Part model, mm, in its own coordinate system. Coordinates: 2 decimals unless noted, no trailing zeros. Order: outer loops, then holes, each group sorted by start corner. A loop starts at its lowest first (then second) coordinate and runs counter-clockwise, first axis right, second up.
from build123d import *

# Parameters (mm, degrees)
SKETCH1_W           = 6.35
SKETCH1_H           = 76.2
BOSS_EXTRUDE1_DEPTH = 114.3
SKETCH2_W           = 6.35
SKETCH2_H           = 50.8
BOSS_EXTRUDE2_DEPTH = 6.35
SKETCH3_W           = 6.35
SKETCH3_H           = 12.7
SKETCH3_W_2         = 95.25
SKETCH3_H_2         = 6.35
SKETCH3_W_3         = 25.4
CUT_EXTRUDE1_DEPTH  = 121.65


with BuildPart() as part:
    # Sketch1 → Boss-Extrude1 (new body)
    with BuildSketch(Plane.XY):
        with Locations((-41.275, 0)):
            Rectangle(SKETCH1_W, SKETCH1_H)
    extrude(amount=BOSS_EXTRUDE1_DEPTH)

    # Sketch2 → Boss-Extrude2 (add, through all)
    with BuildSketch(Plane(origin=(-38.1, 0, 0), x_dir=(0, 0, -1), z_dir=(1, 0, 0))):
        with Locations((3.175, 0)):
            Rectangle(SKETCH2_W, SKETCH2_H)
    extrude(amount=-BOSS_EXTRUDE2_DEPTH)

    # Sketch3 → Cut-Extrude1 (cut, through all)
    with BuildSketch(Plane(origin=(-38.1, 0, 0), x_dir=(0, 0, -1), z_dir=(1, 0, 0))):
        with Locations((-111.125, -31.75)):
            Rectangle(SKETCH3_W, SKETCH3_H)
        with Locations((-111.125, 31.75)):
            Rectangle(SKETCH3_W, SKETCH3_H)
        with Locations((-53.975, 31.75)):
            Rectangle(SKETCH3_W_2, SKETCH3_H_2)
        with Locations((-12.7, -34.925)):
            Rectangle(SKETCH3_W_3, SKETCH3_H_2)
    extrude(amount=-CUT_EXTRUDE1_DEPTH, mode=Mode.SUBTRACT)


solid = part.part
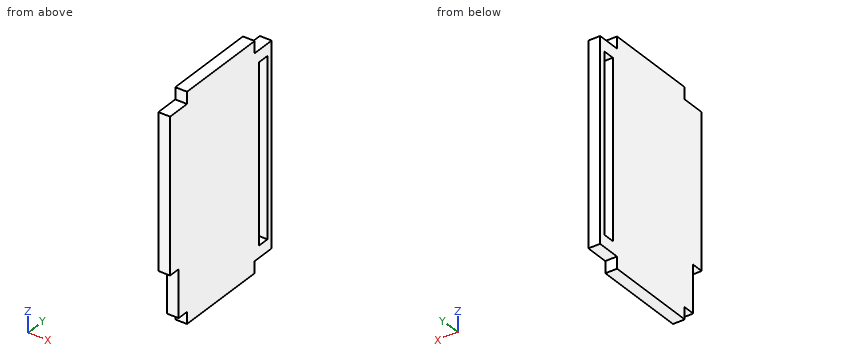
Q1. Cut at C-C on x = -42. Write the cut outline in (y, z) (3 decimals).
Results list:
outline: (-38.1, 25.4) - (-31.75, 25.4) - (-31.75, 0) - (-25.4, 0) - (-25.4, -6.35) - (25.4, -6.35) - (25.4, 0) - (38.1, 0) - (38.1, 107.95) - (25.4, 107.95) - (25.4, 114.3) - (-25.4, 114.3) - (-25.4, 107.95) - (-38.1, 107.95) - close; hole (28.575, 6.35) - (34.925, 6.35) - (34.925, 101.6) - (28.575, 101.6) - close
Q2. Pin check, flat tips, straight feed: pin 1 Ø1.5 at (x, y) = (-43.5, -28.5) entering from +Z; pin 2 Ø1.9 at (x, y) = (-42.5, -29) entering from -Z; pin 3 Ø3 at (x, z) = (-40.5, -2) entering from -Y. Stop position of each tip, or through.
Results list:
pin 1: stops at z = 107.95
pin 2: stops at z = 0
pin 3: stops at y = -25.4
Q3. Wall check: line 1 along Y through (x, z) = (-39.75, 66) (3 decimals); line 2 along Y through (x, z) = (-39.75, 14) (3 decimals); line 3 along Z through (x, y) = (-42, 32). Give the ranges that are in metal, low to high.
Results list:
line 1: y = -38.1 to 28.575, 34.925 to 38.1
line 2: y = -31.75 to 28.575, 34.925 to 38.1
line 3: z = 0 to 6.35, 101.6 to 107.95
Q4. Cut at A-A on y = 30. Write the cut outline in (x, z), and give its area (3 significant figures).
Results list:
outline: (-44.45, 0) - (-38.1, 0) - (-38.1, 6.35) - (-44.45, 6.35) - close; (-44.45, 101.6) - (-38.1, 101.6) - (-38.1, 107.95) - (-44.45, 107.95) - close
area: 80.6 mm2
Q5. Cut at B-B on z = 19. Write the cut outline in (x, y) (3 decimals), and give its area (3 significant figures).
Results list:
outline: (-44.45, -31.75) - (-38.1, -31.75) - (-38.1, 28.575) - (-44.45, 28.575) - close; (-44.45, 34.925) - (-38.1, 34.925) - (-38.1, 38.1) - (-44.45, 38.1) - close
area: 403 mm2
